Autodesk Inventor part; units mm, degrees
ref_plane "YZ Plane" through (0, 0, 0) normal (1, 0, 0) x (0, 1, 0)
ref_plane "XZ Plane" through (0, 0, 0) normal (0, 1, 0) x (-1, 0, 0)
ref_plane "XY Plane" through (0, 0, 0) normal (0, 0, 1) x (1, 0, 0)
sketch "スケッチ1" plane through (0, 0, 0) normal (0, 1, 0) x (-1, 0, 0)
  line L0 (0, 0) -> (-64.0652, 0) construction
  circle A0 centre (-14.1, 0) radius 1.75
  line L1 (-9.1, -2.25) -> (-14.1, -2.25)
  line L2 (-14.1, -2.25) -> (-14.1, 2.25)
  line L3 (-14.1, 2.25) -> (-9.1, 2.25)
  line L4 (-9.1, 2.25) -> (-9.1, -2.25)
  line L5 (0, -4.9) -> (0, 4.9)
  point P0 (-14.1, 1.75)
  point P1 (-14.1, -1.75)
  dimension "P_DIA" = 3.5
  dimension "P_D1" = 14.1
  dimension "WW" = 4.5
  dimension "d3" = 5
revolve "リム" add sketch "スケッチ1" angle 360 about axis through (0, 0, -10) along (0, 0, 1) contours A0 L2 L3 L4 L1
sketch "スケッチ3" plane through (0, 0, 2.25) normal (0, 0, 1) x (1, 0, 0)
  line L0 (-5, 2.8868) -> (0, 5.7735)
  line L1 (0, 5.7735) -> (5, 2.8868)
  line L2 (5, 2.8868) -> (5, -2.8868)
  line L3 (5, -2.8868) -> (0, -5.7735)
  line L4 (0, -5.7735) -> (-5, -2.8868)
  line L5 (-5, -2.8868) -> (-5, 2.8868)
  point P0 (0, 0)
  point P1 (0, 0)
  dimension "HUB_DIA" = 10
extrude "ハブ" add sketch "スケッチ3" against normal up to surface (4.5 mm away)
sketch "スケッチ4" plane through (0, 0, 2.25) normal (0, 0, 1) x (1, 0, 0)
  line L0 (-0.8, 0) -> (0.8, 0)
  line L1 (0.8, 0) -> (0.8, 9.1)
  line L2 (0.8, 9.1) -> (-0.8, 9.1)
  line L3 (-0.8, 9.1) -> (-0.8, 0)
  circle A0 centre (0, 0) radius 9.1
  point P0 (0, 9.1)
  dimension "SPOKE_THIN" = 1.6
extrude "スポーク" add sketch "スケッチ4" against normal up to surface (4.5 mm away) contours L3 A0 L1 L0 | L3 L2 A0 | A0 L2 L1 picked at (0, 3.0333)
pattern_circular "円形状パターン1" count 6 over 360 about axis through (0, 0, -10) along (0, 0, 1) of "スポーク"
sketch "スケッチ5" plane through (0, 0, 2.25) normal (0, 0, 1) x (1, 0, 0)
  line L0 (-2, 1.525) -> (2, 1.525)
  line L1 (2, 1.525) -> (2, -1.525)
  line L2 (2, -1.525) -> (-2, -1.525)
  line L3 (-2, -1.525) -> (-2, 1.525)
  point P0 (0, 0)
  point P1 (0, 1.525)
  point P2 (-2, 0)
  dimension "d15" = 4
  dimension "d16" = 3.05
extrude "軸穴" cut sketch "スケッチ5" against normal through all
properties part number "Wheel-D63C"
Here's how the part is built. I have some questions about the finished solid (model axes, mm). A direction names the side the tool comes from. Round coordinates to 2 decimals unless told otherwise and drop trailing zeros. Order: outer loops, then holes, each group sorted by start corner. A loop starts at its lowest first (then second) coordinate and runs counter-clockwise, first axis right, second up. Notation, with made-up numbers: (7.5, 75) -> (50.5, 75) arc R29 cw to (50.5, 109) -> close; hole circle Ø4 at (70.5, -12.75). An arc over 180 degrees is marked (long way). Use CSV: the item, a comma, the result in double quotes.
1. I want a section at B-B on x = 0. List the corners of the cut face in (y, z) for me (3 decimals).
Recorded:
outline,"(-14.1, -2.25) -> (-1.525, -2.25) -> (-1.525, 2.25) -> (-14.1, 2.25) -> (-14.1, 1.75) arc R1.75 cw to (-14.1, -1.75) -> close; (1.525, -2.25) -> (14.1, -2.25) -> (14.1, -1.75) arc R1.75 cw to (14.1, 1.75) -> (14.1, 2.25) -> (1.525, 2.25) -> close"
2. I'm going to push flat-ended pins straight in: P1, Ø1.5, axis at y = 0, z = 0, coming from the +X side; P2, Ø1.2, axis at x = 0, z = 0, coming from the -Y side; P3, Ø2, axis at y = -0.5, z = 0, coming from the +X side (3 decimals). Where does each tip first touch, or does it pass through?
Recorded:
P1,"stops at x = 12.52"
P2,"stops at y = -12.46"
P3,"stops at x = 12.655"
3. I want a section at C-C on z = 0. Give the number of separate pieces and of enclosed holes in the cut face, and give its area (3 significant figures).
Recorded:
separate pieces,"1"
enclosed holes,"7"
area,"327 mm2"
4. I need wall thicknesses on line 1 along Z through (x, y) = (-9.25, 10.5); line 2 along X through (y, z) = (-5.5, 0.75); line 3 along X through (y, z) = (-1, -1.2). Which ranges of each line are inside material? Lowest first, please.
Recorded:
line 1,"z = -2.25 to -1.75, 1.75 to 2.25"
line 2,"x = -11.25 to -7.25, -0.8 to 0.8, 7.25 to 11.25"
line 3,"x = -12.79 to -9.04, -5 to -2, 2 to 5, 9.04 to 12.79"
5. Which directions (+Z, -Z, +X, -X, +Y, -Y) give clear straight access to the entire face, cutting with the end or side of a thin tool? Please do faces 3 (the face through (3, 0, -2.25)), 4 (the face through (0.8, -7, 0)).
Recorded:
face 3,"-Z, +X, -X, +Y, -Y"
face 4,"+Z, -Z"
6. Thinking about a two-plate mould opening in Y: for faces 1 (the face through (-0.8, -7, 0)), 2 (the face through (3, 0, 2.25)), which applies, pulls with the +Y half, pulls with the -Y half, needs draft (parallel to the pull), parting line crosses it, or undercut?
Recorded:
face 1,"undercut"
face 2,"needs draft"
7. I want a section at A-A on y = 0. List the corners of the cut face in (x, z) for me.
Recorded:
outline,"(-14.1, -2.25) -> (-9.1, -2.25) -> (-9.1, 2.25) -> (-14.1, 2.25) -> (-14.1, 1.75) arc R1.75 cw to (-14.1, -1.75) -> close; (-5, -2.25) -> (-2, -2.25) -> (-2, 2.25) -> (-5, 2.25) -> close; (2, -2.25) -> (5, -2.25) -> (5, 2.25) -> (2, 2.25) -> close; (9.1, -2.25) -> (14.1, -2.25) -> (14.1, -1.75) arc R1.75 cw to (14.1, 1.75) -> (14.1, 2.25) -> (9.1, 2.25) -> close"
